Part print with two shaded views. Sizes in mm from the minimum x, y, z corner. Give positions to 0.01 mm unless a question says otherwise; leave off trailing zeros. Order: outer loops, then holes, each group sorted by start corner. A loop starts at its lowest first (then second) coordinate and runs counter-clockwise, first axis right, second up. Notation, with made-up numbers: M -35.5,24 L -0.5,24 A26 ccw -0.5,63 Z; hole C -8.75,62 d5. An arc over 180 degrees is marked long. Return JSON: item names as keys, results as strings.
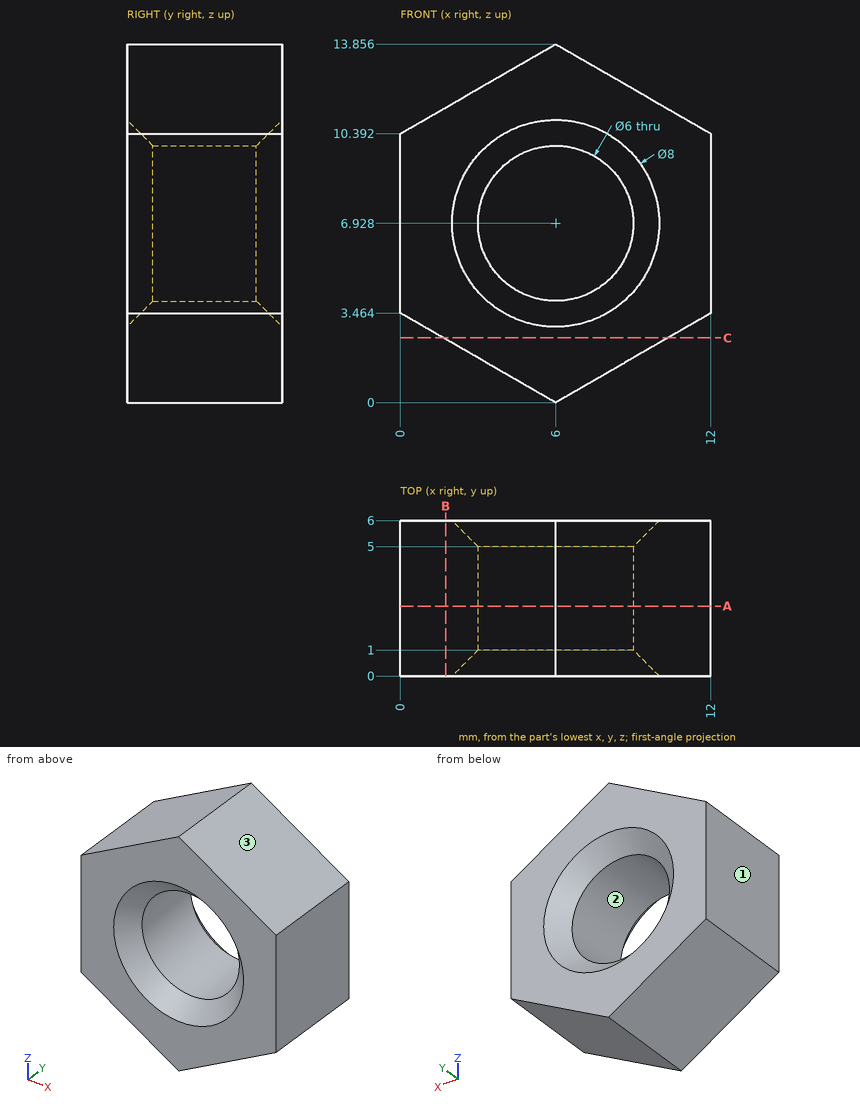
Q1. Band-saw the part on B-B (x = 1.75). Give the cut face in (y, z), then the cut area to 3 significant figures.
Established:
{"outline": "M 0,2.45 L 6,2.45 L 6,11.4 L 0,11.4 Z", "area": "53.7 mm²"}
Q2. Band-saw the part on C-C (z = 2.5). Give the cut face in (x, y).
Established:
{"outline": "M 1.67,0 L 10.33,0 L 10.33,6 L 1.67,6 Z"}
Q3. Probe line 1 along Z through (x, y) = (5.5, 1.7) (1 decimal); line 2 along X through (y, z) = (3.65, 4.75) (1 decimal); line 3 along X through (y, z) = (4.8, 6.5). List the from-to ranges inside material, lowest first.
Established:
{"line 1": "z = 0.3 to 4, 9.9 to 13.6", "line 2": "x = 0 to 3.9, 8.1 to 12", "line 3": "x = 0 to 3.03, 8.97 to 12"}
Q4. Band-saw the part on A-A (y = 2.7). Give the cut face in (x, z).
Established:
{"outline": "M 0,3.46 L 6,0 L 12,3.46 L 12,10.39 L 6,13.86 L 0,10.39 Z; hole C 6,6.93 d6"}
Q5. Two-plate mould, pull along X, no slides. Class the marked faces 1, 2 and 3: +X half, -X half, draft (parallel to the pull), parting line (faces both ways), or undercut.
Established:
{"face 1": "-X half", "face 2": "undercut", "face 3": "+X half"}
Q6. Pin check, flat tip, straight feed: pin 1 (1 mm diameter, centred on x = 8.5, z = 9, fed in from -Y). Stop position of the tip, or through.
Established:
{"pin 1": "stops at y = 0.25"}
